from build123d import *

# Parameters (mm, degrees)
BOSS_EXTRUDE1_DEPTH = 25.4
SKETCH2_W           = 38.1
SKETCH2_H           = 38.1
CUT_EXTRUDE1_DEPTH  = 12.7
SKETCH3_R           = 4.191
CUT_EXTRUDE2_DEPTH  = 314.875552812
SKETCH4_R           = 4.191
CUT_EXTRUDE3_DEPTH  = 25.4
FILLET1_R           = 6.35
FILLET2_R           = 3.175


with BuildPart() as part:
    # Sketch1 → Boss-Extrude1 (new body)
    with BuildSketch(Plane.XY):
        Polygon((0, 0), (0, 12.7), (50.8, 12.7), (88.9, -20.510228633), (152.4, -260.515926793), (38.018659419, -260.515926793), (38.018659419, -190.696503564), (30.48, -85.763926793), (0, -85.763926793), (0, -73.152260366), (38.018659419, -73.152260366), (38.018659419, 0), align=None)
    extrude(amount=BOSS_EXTRUDE1_DEPTH)

    # Sketch2 → Cut-Extrude1 (cut)
    with BuildSketch(Plane(origin=(0, 0, 0), x_dir=(-1, 0, 0), z_dir=(0, 0, -1))):
        with Locations((-82.468659419, -163.487926793)):
            Rectangle(SKETCH2_W, SKETCH2_H)
    extrude(amount=-CUT_EXTRUDE1_DEPTH, mode=Mode.SUBTRACT)

    # Sketch3 → Cut-Extrude2 (cut, through all)
    with BuildSketch(Plane(origin=(0, 12.7, 0), x_dir=(1, 0, 0), z_dir=(0, 1, 0))):
        with Locations(Location((11.684, -12.7, 0), (0, 0, 270))):
            Circle(SKETCH3_R)
    extrude(amount=-CUT_EXTRUDE2_DEPTH, mode=Mode.SUBTRACT)

    # Sketch4 → Cut-Extrude3 (cut)
    with BuildSketch(Plane(origin=(0, -260.515926793, 0), x_dir=(-1, 0, 0), z_dir=(0, -1, 0))):
        with Locations(Location((-139.7, -12.7, 0), (0, 0, 180))):
            Circle(SKETCH4_R)
        with Locations(Location((-63.5, -11.81655653, 0), (0, 0, 180))):
            Circle(SKETCH4_R)
    extrude(amount=-CUT_EXTRUDE3_DEPTH, mode=Mode.SUBTRACT)

    # Fillet1
    # the kernel refuses this fillet: 6.35 mm, written as the material it adds along each edge
    with BuildSketch(Plane(origin=(38.018659419, -190.696503564, 0), x_dir=(0, -1, 0), z_dir=(0, 0, 1))) as fillet1_piece_1:
        with BuildLine():
            CenterArc((FILLET1_R * 0.0358752122725, -FILLET1_R), FILLET1_R, 90, 4.109234206)
            Line((-FILLET1_R * 0.0357829859603, -FILLET1_R * 0.00257075307266), (0, 0))
            Line((0, 0), (FILLET1_R * 0.0358752122725, 0))
        make_face()
    extrude(amount=25.4)
    # the kernel refuses this fillet: 6.35 mm, written as the material it takes off along each edge
    with BuildSketch(Plane(origin=(50.8, 12.7, -5.947635314), x_dir=(-1, 0, 0), z_dir=(0, 0, 1))) as fillet1_2_piece_1:
        with BuildLine():
            CenterArc((FILLET1_R * 0.374654193004, FILLET1_R), FILLET1_R, 228.922654606, 41.077345394)
            Line((-FILLET1_R * 0.282423044355, FILLET1_R * 0.246176742103), (0, 0))
            Line((0, 0), (FILLET1_R * 0.374654193004, 0))
        make_face()
    extrude(amount=37.295270628, mode=Mode.SUBTRACT)
    with BuildSketch(Plane(origin=(88.9, -20.510228633, -4.869092834), x_dir=(-0.7538232578965339, 0.6570772373581782, 0), z_dir=(0, 0, 1))) as fillet1_2_piece_2:
        with BuildLine():
            CenterArc((FILLET1_R * 0.306714509228, FILLET1_R), FILLET1_R, 235.896927034, 34.103072966)
            Line((-FILLET1_R * 0.253968896194, FILLET1_R * 0.171969735526), (0, 0))
            Line((0, 0), (FILLET1_R * 0.306714509228, 0))
        make_face()
    extrude(amount=35.138185668, mode=Mode.SUBTRACT)

    # Fillet2
    fillet2_edges = [part.edges().sort_by_distance(p)[0] for p in [
        (101.518659419, -182.537926793, 6.35),
        (101.518659419, -144.437926793, 6.35),
        (63.418659419, -144.437926793, 6.35),
        (63.418659419, -182.537926793, 6.35),
    ]]
    fillet(fillet2_edges, radius=FILLET2_R)


solid = part.part
Can you work these out from the model? Positions are in its coordinate system, mm. A direction names the side the tool comes from. Give positions to 0.01 mm unless a question says otherwise; leave off trailing zeros. Loops run counter-clockwise (first coordinate to the right, second up) from the corner with the lowest first, then second, coordinate; pieces in that order, holes last. Notation, with made-up numbers: (25, 15) - (71, 15) arc R35 ccw to (71, 49) - close; hole circle Ø5 at (-1.75, 59). An arc over 180 degrees is marked (long way). Answer as a JSON object with one key per item and string values.
Q1. If I drill on L1, parallel to Z at x = 63.5, y = -250; L2, parallel to Z at x = 139.7, y = -253.75; L3, parallel to X at y = -182, z = 1, over which ranges is the centre line in solid material (lowest first)?
Geometry says:
{"L1": "0 to 7.63, 16.01 to 25.4", "L2": "0 to 8.51, 16.89 to 25.4", "L3": "37.39 to 64.83, 100.11 to 131.63"}
Q2. If we mould it in two halves opening along Z, with no side actions, what happens to faces 4 (the cylindrical face through (135.513, -247.994, 12.884)), 5 (the flat face through (0, -80, 13)), 6 (the flat face through (83, -163, 12.7))? For each: pulls with the +Z half, pulls with the -Z half, needs draft (parallel to the pull), parting line crosses it, or undercut.
Geometry says:
{"face 4": "undercut", "face 5": "needs draft", "face 6": "pulls with the -Z half"}
Q3. Which directions (+Z, -Z, +X, -X, +Y, -Y) give clear straight access to the entire face, cutting with the end or side of a thin tool? Please do faces 1 (the flat face through (19, -73.152, 13)), 2 (the flat face through (83, -182.538, 6)), 3 (the flat face through (140, -235.116, 13)).
Geometry says:
{"face 1": "+Z, -Z, -X", "face 2": "-Z", "face 3": "-Y"}
Q4. Imagine slicing it at C-C on y = -99. Write out the boundary of the cut face in (x, z), plus the area to 3 significant figures.
Geometry says:
{"outline": "(31.43, 0) - (109.67, 0) - (109.67, 25.4) - (31.43, 25.4) - close", "area": "1,990 mm²"}
Q5. Imagine slicing it at A-A on x = 139.7. Write out the boundary of the cut face in (y, z).
Geometry says:
{"outline": "(-260.52, 0) - (-212.51, 0) - (-212.51, 25.4) - (-260.52, 25.4) - (-260.52, 16.89) - (-235.12, 16.89) - (-235.12, 8.51) - (-260.52, 8.51) - close"}
Q6. Will these pins go through, and if not, where does the flat tip stop? P1, Ø10, axis at y = -164.5, z = 5, coming from the +X side; P2, Ø12, axis at x = 61, z = 14.5, coming from the +Y side; P3, Ø11, axis at x = 63.5, z = 11.82, coming from the +Y side; P4, Ø11, axis at x = 11.684, z = 12.7, coming from the +Y side.
Geometry says:
{"P1": "x = 128.32", "P2": "y = 9.04", "P3": "y = 6.42", "P4": "y = 12.7"}
Q7. Imagine slicing it at B-B on y = -205.5. Write out the boundary of the cut face in (x, z), plus the area to 3 significant figures.
Geometry says:
{"outline": "(38.02, 0) - (137.84, 0) - (137.84, 25.4) - (38.02, 25.4) - close", "area": "2,540 mm²"}
